from build123d import *

# Parameters (mm, degrees)
F0_R     = 76.2
F0_R_2   = 69.85
F1_DEPTH = 25.4
F2_DEPTH = 76.2
F3_R     = 70.0511515775
F4_DEPTH = 6.35
F6_DEPTH = 25.4


with BuildPart() as f1:
    # F0 (on Front) → F1 (new body)
    with BuildSketch(Plane.XZ):
        Circle(F0_R)
        Circle(F0_R_2, mode=Mode.SUBTRACT)
    extrude(amount=F1_DEPTH)

    # F2 (add): a face of the model
    f2_faces = [f1.faces().sort_by_distance(p)[0] for p in [
        (-74.0447385309, -25.4, 0),
    ]]
    extrude(f2_faces, amount=F2_DEPTH)

    # F3 (on Front) → F4 (join)
    with BuildSketch(Plane.XZ):
        Circle(F3_R)
    extrude(amount=F4_DEPTH)

    # F5 (on Right) → F6 (join)
    with BuildSketch(Plane.YZ):
        with BuildLine():
            add(Edge.make_bspline(
                [(-27.6209320873, 52.8044328094), (-19.1718805943, 63.260073286), (113.9909728332, 64.3613693038), (44.95583544, 16.606444594), (-34.7977200102, 43.9232093535), (-27.6209320873, 52.8044328094)],
                knots=[0, 0, 0, 0, 0.4070795235, 0.6542187711, 1, 1, 1, 1], degree=3))
        make_face()
    extrude(amount=F6_DEPTH)


solid = f1.part
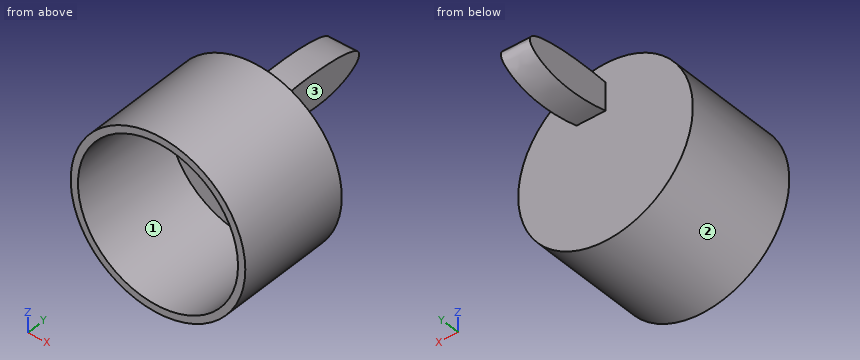
Here's how the part is built. I have some questions about the finished solid (model axes, mm). Face numbers are marked on the shaded views. Give positions to 0.01 mm unless a question says otherwise; leave off trailing zeros. Loops run counter-clockwise (first coordinate to the right, second up) from the corner with the lowest first, then second, coordinate; pieces in that order, holes last. Notation, with made-up numbers: (8.25, 26.5) -> (30.25, 26.5) arc R18 cw to (30.25, 56.5) -> close; hole circle Ø5 at (-25, -20.75). An arc over 180 degrees is marked (long way). Answer as a JSON object with one key per item and string values. Group by question number.
Item 1: Imagine slicing it at A-A on z = 0. Write out the boundary of the cut face in (x, y).
Item 2: Thinking about a two-plate mould opening in Z: for the marked faces 1, 2 and 3, which applies, pulls with the +Z half, pulls with the -Z half, needs draft (parallel to the pull), parting line crosses it, or undercut?
Item 3: Will these pins go through, and if not, where does the flat tip stop? pin 1 (2 mm diameter, centred on y = -48, z = 6.5, fed in from +X); pin 2 (8 mm diameter, centred on y = -77, z = -57.5, fed in from +X); pin 3 (1 mm diameter, centred on y = -62, z = -3, fed in from -X).
Item 4: Imagine slicing it at B-B on x = -61. Write out the boundary of the cut face in (y, z), then the cut area to 3 significant figures.
Item 5: I need wall thicknesses on L1, parallel to Z at x = 0, y = -71; L2, parallel to Z at x = 20.5, y = -27; L3, parallel to Y at x = -50.5, z = -15. Which ranges of each line are inside material? Lowest first, please.
Item 6: Imagine slicing it at C-C on y = -89.5. Write out the boundary of the cut face in (x, z), then the cut area to 3 significant figures.
Answer list:
{
 "1": {"outline": "(-76.2, -101.6) -> (-69.85, -101.6) -> (-69.85, -6.35) -> (69.85, -6.35) -> (69.85, -101.6) -> (76.2, -101.6) -> (76.2, 0) -> (-76.2, 0) -> close"},
 "2": {"face 1": "undercut", "face 2": "parting line crosses it", "face 3": "needs draft"},
 "3": {"pin 1": "stops at x = 76", "pin 2": "stops at x = 54.26", "pin 3": "stops at x = -76.16"},
 "4": {"outline": "(-101.6, -45.67) -> (0, -45.67) -> (0, 45.67) -> (-101.6, 45.67) -> (-101.6, 34.03) -> (-6.35, 34.03) -> (-6.35, -34.03) -> (-101.6, -34.03) -> close", "area": "2,800 mm2"},
 "5": {"L1": "z = -76.2 to -69.85, 69.85 to 76.2", "L2": "z = -73.39 to -66.77, 47.84 to 53.44, 66.77 to 73.39", "L3": "y = -6.35 to 0"},
 "6": {"outline": "circle Ø152.4 at (0, 0); hole circle Ø139.7 at (0, 0)", "area": "2,910 mm2"}
}
